The model under review builds one solid part; all positions refer to its coordinate system, in mm. A direction names the side the tool comes from. Give positions to 0.01 mm unless a question says otherwise; leave off trailing zeros. Loops run counter-clockwise (first coordinate to the right, second up) from the corner with the lowest first, then second, coordinate; pieces in that order, holes last. Notation, with made-up numbers: M 19.25,-7 L 66.25,-7 A35 ccw 66.25,30 Z; hole C -2,32.25 d6. An arc over 180 degrees is marked long. Return JSON: item names as keys, results as strings.
```python
from build123d import *

# Parameters (mm, degrees)
SKETCH1_R          = 3.3909
BASE_FLANGE1_DEPTH = 3.175
EDGE_FLANGE1_DEPTH = 25.4
FILLET1_R          = 3.175
HOLE2_START        = -57.15
HOLE2_OUTLINE_R    = 3.3909
HOLE2_DEPTH        = 3.175
CUT_EXTRUDE1_DEPTH = 48.842508784


# Read off the part's stored shape, not the designer's step: Hole2
# Sheet-metal steps are written as plain solids
with BuildPart() as part:
    # Sketch1 → Base-Flange1 (new body)
    with BuildSketch(Plane(origin=(0, 0, 0), x_dir=(1, 0, 0), z_dir=(0, 1, 0))):
        with BuildLine():
            Line((-12.7, 50.8), (12.7, 50.8))
            Line((12.7, 50.8), (7.700506095, 30.80202438))
            ThreePointArc((7.700506095, 30.80202438), (0, 31.75), (-7.700506095, 30.80202438))
            Line((-7.700506095, 30.80202438), (-12.7, 50.8))
        make_face()
        with Locations(Location((0, 41.91, 0), (0, 0, 270))):
            Circle(SKETCH1_R, mode=Mode.SUBTRACT)
    extrude(amount=-BASE_FLANGE1_DEPTH)

    # Edge-Flange1 section (across the edge) → Edge-Flange1 (add)
    with BuildSketch(Plane(origin=(12.7, 0, -53.975), x_dir=(0, 0, 1), z_dir=(-1, 0, 0))):
        with BuildLine():
            Line((-3.175, 3.175), (-3.175, 38.227))
            Line((-3.175, 38.227), (0, 38.227))
            Line((0, 38.227), (0, 3.175))
            ThreePointArc((0, 3.175), (0.92993597, 0.92993597), (3.175, 0))
            Line((3.175, 0), (3.175, -3.175))
            ThreePointArc((3.175, -3.175), (-1.315128061, -1.315128061), (-3.175, 3.175))
        make_face()
    extrude(amount=EDGE_FLANGE1_DEPTH)

    # Fillet1
    fillet1_edges = [part.edges().sort_by_distance(p)[0] for p in [
        (7.700506095, -1.5875, -30.80202438),
        (-7.700506095, -1.5875, -30.80202438),
    ]]
    fillet(fillet1_edges, radius=FILLET1_R)

    # Hole2 outline → Hole2 (cut)
    with BuildSketch(Plane.XY.offset(HOLE2_START)):
        with Locations((0, 25.4)):
            Circle(HOLE2_OUTLINE_R)
    extrude(amount=HOLE2_DEPTH, mode=Mode.SUBTRACT)

    # Sketch11 → Cut-Extrude1 (cut, through all)
    with BuildSketch(Plane(origin=(0, 0, -57.15), x_dir=(-1, 0, 0), z_dir=(0, 0, -1))):
        with BuildLine():
            Line((-12.7, 25.4), (-12.7, 38.227))
            Line((-12.7, 38.227), (12.7, 38.227))
            Line((12.7, 38.227), (12.7, 25.4))
            ThreePointArc((12.7, 25.4), (0, 38.1), (-12.7, 25.4))
        make_face()
    extrude(amount=-CUT_EXTRUDE1_DEPTH, mode=Mode.SUBTRACT)


solid = part.part
```
1) Insertion check: pin 1 (1.5 mm diameter, centred on x = -4, z = -41.5, fed in from +Y); pin 2 (4 mm diameter, centred on x = 0, z = -41.91, fed in from -Y). Each pin has a flat end and moves straight along its axis. Give the tip position at first contact, or say it passes through.
From the geometry:
{"pin 1": "y = 0", "pin 2": "through"}
2) The part is to be moulded in two halves that separate along X. For faces 3 (the face through (0.07, -1.57, -31.75)), 4 (the face through (0.178, -1.364, -55.24)), 5 (the face through (-10.538, -1.565, -42.152)), say which applies: released by +X, released by -X, zero draft, split by the parting line, or undercut.
From the geometry:
{"face 3": "undercut", "face 4": "zero draft", "face 5": "released by -X"}
3) Consider section C-C on y = 10. Write out the cut boundary in (x, z) (3 decimals), then the cut area to 3 significant figures.
From the geometry:
{"outline": "M -12.7,-57.15 L 12.7,-57.15 L 12.7,-53.975 L -12.7,-53.975 Z", "area": "80.6 mm²"}
4) Consider section A-A on x = 0. Write out the cut boundary in (y, z) (3 decimals), then the cut area to 3 significant figures.
From the geometry:
{"outline": "M -3.175,-50.8 A6.35 ccw 3.175,-57.15 L 22.009,-57.15 L 22.009,-53.975 L 3.175,-53.975 A3.175 cw 0,-50.8 L 0,-45.301 L -3.175,-45.301 Z; M -3.175,-38.519 L 0,-38.519 L 0,-31.75 L -3.175,-31.75 Z; M 28.791,-57.15 L 38.1,-57.15 L 38.1,-53.975 L 28.791,-53.975 Z", "area": "152 mm²"}
5) Consider section D-D on x = 11.25. Write out the cut boundary in (y, z) (3 decimals).
From the geometry:
{"outline": "M -3.175,-50.8 A6.35 ccw 3.175,-57.15 L 31.293,-57.15 L 31.293,-53.975 L 3.175,-53.975 A3.175 cw 0,-50.8 L 0,-45 L -3.175,-45 Z"}
6) Wall thickness on L1, parallel to Z at x = 5.25, y = 13 (3 decimals); L2, parallel to Y at x = -4.75, z = -38 (3 decimals); L3, parallel to X at y = -1, z = -41.91: over which ranges is each line inside the solid? List them lowest first. Write a range as from..to.
From the geometry:
{"L1": "-57.15..-53.975", "L2": "-3.175..0", "L3": "-10.48..-3.39, 3.39..10.48"}
7) Consider section B-B on z = -43.5. Write out the cut boundary in (x, y) (3 decimals), then the cut area to 3 significant figures.
From the geometry:
{"outline": "M -10.875,-3.175 L -2.995,-3.175 L -2.995,0 L -10.875,0 Z; M 2.995,-3.175 L 10.875,-3.175 L 10.875,0 L 2.995,0 Z", "area": "50.0 mm²"}
8) Tool access review of faces 1 (the face through (0, 0, -46)), 2 (the face through (-12.7, 11, -55)): name each direction out of +Z, -Z, +X, -X, +Y, -Y from which nothing blocks a thin tool from reaching the whole face with its end or side.
From the geometry:
{"face 1": "+Z, +X, -X, +Y", "face 2": "+Z, -Z, -X, +Y, -Y"}
